from build123d import *

# Parameters (mm, degrees)
SKETCH_2_R               = 1.2
CUT_EXTRUDE_1_DEPTH      = 8
PATTERN_CIRCULAR_1_COUNT = 8
SKETCH_3_R               = 1.55
CUT_EXTRUDE_2_DEPTH      = 10


with BuildPart() as part:
    # 草图1 → 旋转1 (revolve)
    with BuildSketch(Plane.XY):
        Polygon((-16, 0), (-17, 0), (-17, 2), (-21, 2), (-21, 6), (-17.5, 8.020725942), (-17.5, 27), (-6.75, 27), (-6.75, 25), (-16, 25), align=None)
    revolve(axis=Axis((0, 0, 0), (0, 1, 0)))

    # 草图2 → 切除-拉伸1 (cut)
    with BuildSketch(Plane.XZ.offset(-2)):
        with Locations((0, -19)):
            Circle(SKETCH_2_R)
    cut_extrude_1 = extrude(amount=-CUT_EXTRUDE_1_DEPTH, mode=Mode.SUBTRACT)

    # 阵列(圆周)1: 切除-拉伸1 ×8 about axis
    pattern_circular_1_axis = Axis((0, 0, 0), (0, 1, 0))
    for i in range(1, PATTERN_CIRCULAR_1_COUNT):
        add(cut_extrude_1.rotate(pattern_circular_1_axis, i * 360 / PATTERN_CIRCULAR_1_COUNT), mode=Mode.SUBTRACT)

    # 草图3 → 切除-拉伸2 (cut)
    with BuildSketch(Plane(origin=(0, 27, 0), x_dir=(1, 0, 0), z_dir=(0, 1, 0))):
        with Locations((0, -9.5)):
            Circle(SKETCH_3_R)
        with Locations((-8.227241336, 4.75)):
            Circle(SKETCH_3_R)
        with Locations((8.227241336, 4.75)):
            Circle(SKETCH_3_R)
    extrude(amount=-CUT_EXTRUDE_2_DEPTH, mode=Mode.SUBTRACT)


solid = part.part
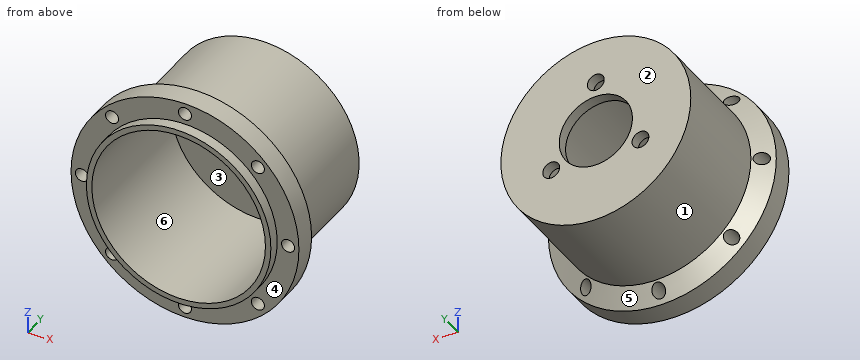
Work out the finished part from the listing and answer in its coordinate system (mm). Face numbers are marked on the shaded views. A direction names the side the tool comes from. Coordinates: 2 decimals unless noted, no trailing zeros. Order: outer loops, then holes, each group sorted by start corner. A loop starts at its lowest first (then second) coordinate and runs counter-clockwise, first axis right, second up. Notation, with made-up numbers: (-22.75, -4.75) - (-6.75, -4.75) arc R36 ccw to (-6.75, 34.25) - close; hole circle Ø5 at (-26.75, 25.25). An arc over 180 degrees is marked (long way). Put each result on its own line as item: value. Start each with the question number.
1) For a pull along Z with two mould halves and no side action, classify the marked faces 4, 5 and 6 as released by +Z, released by -Z, zero draft, split by the parting line, or undercut.
2) Find section B-B (y = 10.25). Give the vertices of the cut face in (x, z), plus the area to 3 significant figures.
3) Find section A-A (x = 0). State how many separate pieces and enclosed holes the cut face has, plus the area to 3 significant figures.
4) Flat-ended cylindrical pins translate along their axes: pin 1 (3 mm diameter, centred on y = 6, z = -10.5, fed in from +X); pin 2 (4 mm diameter, centred on x = 1.5, y = 10.5, fed in from -Z); pin 3 (3 mm diameter, centred on x = 0, z = 19, fed in from -Y). Find the tip coordinate at first contact, or state that the pin passes through.
5) Find the intervals of material crossed by line 1 (Z direction, x = 0, y = 3.45); line 2 (Y direction, x = -12.5, z = -3); line 3 (Y direction, x = -6, z = -16), in increasing order. Write a range as from..to.
6) For the marked faces 1, 2 and 3, determine the directions among +Z, -Z, +X, -X, +Y, -Y from which every point of the face is accessible in a straight line to the end or side of a thin tool.
Results list:
1. face 4: zero draft
1. face 5: split by the parting line
1. face 6: undercut
2. outline: circle Ø35 at (0, 0); hole circle Ø32 at (0, 0)
2. area: 158 mm^2
3. separate pieces: 5
3. enclosed holes: 0
3. area: 120 mm^2
4. pin 1: stops at x = 18.97
4. pin 2: stops at z = -17.5
4. pin 3: stops at y = 2
5. line 1: z = -21..-20.2, -17.8..-16, 16..17.8, 20.2..21
5. line 2: y = 25..27
5. line 3: y = 2..27
6. face 1: +Y
6. face 2: +Z, -Z, +X, -X, +Y
6. face 3: -Y
